Build history of the part. All positions in model axes, mm. Face numbers are marked on the shaded views. A direction names the side the tool comes from. Give positions to 0.01 mm unless a question says otherwise; leave off trailing zeros. Write each loop counter-clockwise with the first axis right and the second up, starting at its lowest first coordinate (ties: lowest second). Pieces come first, ordered by that corner, then holes. Notation, with made-up numbers: (-22, 48.25) -> (11, 48.25) arc R21 ccw to (11, 86.25) -> close; hole circle Ø3 at (54.5, 5.5). An arc over 180 degrees is marked (long way). Put each result on its own line as item: value. Start each with the question number.
Item 1: Drill centre lines: line 1 along Y through (x, z) = (-94.5, -1.75); line 2 along X through (y, z) = (137.5, -2); line 3 along Y through (x, z) = (4, -16.5). Where is each one in solid material? Low to high.
Item 2: Slice it at A-A, the plane x = 200.5. List the corners of the cut face in (y, z).
Item 3: Slice it at B-B, the plane y = 218. List the corners of the cut face in (x, z).
Item 4: Tool access for the marked faces 1 and 2: list every direction of +Z, -Z, +X, -X, +Y, -Y with a clear straight run to the whole face (end or side of a thin tool).
Item 5: Flat gauge pins, fed straight in: pin 1 Ø8 at (x, z) = (-129.5, -5.5) entering from -Y; pin 2 Ø19 at (x, y) = (-238.16, 137.5) entering from -Z; pin 3 Ø10 at (x, z) = (6.5, -17.5) entering from +Y. Where does each tip first touch, or does it go through?
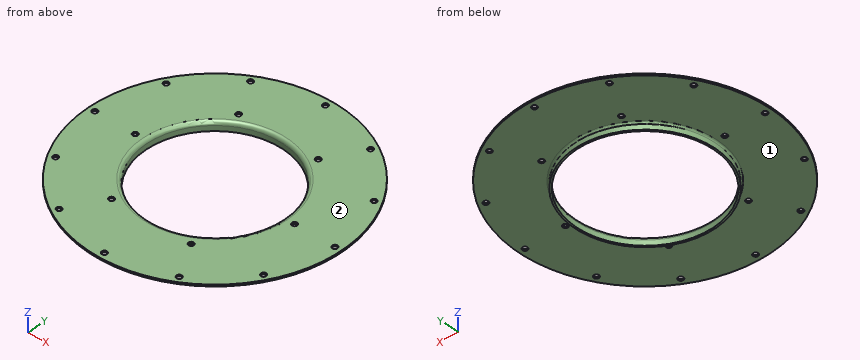
```python
from build123d import *

# Parameters (mm, degrees)
SKETCH2_R          = 6
CUT_EXTRUDE1_DEPTH = 10
CIRPATTERN1_COUNT  = 6
SKETCH3_R          = 6
CUT_EXTRUDE2_DEPTH = 10
CIRPATTERN2_COUNT  = 12


with BuildPart() as part:
    # Sketch1 → Revolve1 (revolve)
    with BuildSketch(Plane(origin=(0, 0, 0), x_dir=(1, 0, 0), z_dir=(0, 1, 0))):
        with BuildLine():
            Line((-161.5, 8), (-161.5, 20))
            Line((-161.5, 20), (-157.5, 20))
            Line((-157.5, 20), (-157.5, 8))
            ThreePointArc((-157.5, 8), (-159.843145751, 2.343145751), (-165.5, 0))
            Line((-165.5, 0), (-290, 0))
            Line((-290, 0), (-290, 4))
            Line((-290, 4), (-165.5, 4))
            ThreePointArc((-165.5, 4), (-162.671572875, 5.171572875), (-161.5, 8))
        make_face()
    revolve(axis=Axis((0, 0, 0), (0, 0, 1)))

    # Sketch2 → Cut-Extrude1 (cut)
    with BuildSketch(Plane.XY):
        with Locations((182.5, 0)):
            Circle(SKETCH2_R)
    cut_extrude1 = extrude(amount=-CUT_EXTRUDE1_DEPTH, mode=Mode.SUBTRACT)

    # CirPattern1: Cut-Extrude1 ×6 about axis
    cirpattern1_axis = Axis((0, 0, 0), (0, 0, 1))
    for i in range(1, CIRPATTERN1_COUNT):
        add(cut_extrude1.rotate(cirpattern1_axis, i * 360 / CIRPATTERN1_COUNT), mode=Mode.SUBTRACT)

    # Sketch3 → Cut-Extrude2 (cut)
    with BuildSketch(Plane.XY):
        with Locations((275, 0)):
            Circle(SKETCH3_R)
    cut_extrude2 = extrude(amount=-CUT_EXTRUDE2_DEPTH, mode=Mode.SUBTRACT)

    # CirPattern2: Cut-Extrude2 ×12 about axis
    cirpattern2_axis = Axis((0, 0, 0), (0, 0, 1))
    for i in range(1, CIRPATTERN2_COUNT):
        add(cut_extrude2.rotate(cirpattern2_axis, i * 360 / CIRPATTERN2_COUNT), mode=Mode.SUBTRACT)


solid = part.part
```
Values follow:
1. line 1: -274.17 to -163.09, -153.01 to -129.74, 129.74 to 153.01, 163.09 to 274.17
1. line 2: -255.33 to -244.16, -232.16 to -82.22, 82.22 to 232.16, 244.16 to 255.33
1. line 3: -161.45 to -157.45, 157.45 to 161.45
2. outline: (-209.52, -4) -> (209.52, -4) -> (209.52, 0) -> (-209.52, 0) -> close
3. outline: (-191.25, -4) -> (191.25, -4) -> (191.25, 0) -> (-191.25, 0) -> close
4. face 1: -Z
4. face 2: +Z, +X, -X, +Y, -Y
5. pin 1: y = -261.3
5. pin 2: z = -4
5. pin 3: y = 161.49
